```python
from build123d import *

# Parameters (mm, degrees)
CYLINDER016_R     = 2
CYLINDER016_DEPTH = 94
CYLINDER030_R     = 2
CYLINDER030_DEPTH = 10
CYLINDER029_R     = 2
CYLINDER029_DEPTH = 10
CYLINDER001_W     = 10
CYLINDER001_H     = 5
CYLINDER001_ANGLE = 90
BOX002_W          = 10
BOX002_H          = 54
BOX002_DEPTH      = 11
BOX001_W          = 10
BOX001_H          = 62
BOX001_DEPTH      = 11
BOX_W             = 10
BOX_H             = 72
BOX_DEPTH         = 25
CYLINDER_W        = 10
CYLINDER_H        = 5
CYLINDER_ANGLE    = 90
CYLINDER017_W     = 10
CYLINDER017_H     = 87
CYLINDER017_ANGLE = 90
BOX004_W          = 25
BOX004_H          = 72
BOX004_DEPTH      = 15


with BuildPart() as obj1:
    # Cylinder016 → Cylinder016 (new body)
    with BuildSketch(Plane(origin=(6, -47.35, 51), x_dir=(1, 0, 0), z_dir=(0, 1, 0))):
        Circle(CYLINDER016_R)
    extrude(amount=CYLINDER016_DEPTH)


with BuildPart() as m3cuts003:
    # Cylinder030 → Cylinder030 (new body)
    with BuildSketch(Plane(origin=(5, 9, 70), x_dir=(1, 0, 0), z_dir=(0, 0, 1))):
        Circle(CYLINDER030_R)
    extrude(amount=CYLINDER030_DEPTH)


with BuildPart() as m3cute001:
    # Cylinder029 → Cylinder029 (new body)
    with BuildSketch(Plane(origin=(5, -9, 70), x_dir=(1, 0, 0), z_dir=(0, 0, 1))):
        Circle(CYLINDER029_R)
    extrude(amount=CYLINDER029_DEPTH)

    # Fusion012: union m3Cuts003
    add(m3cuts003.part)


with BuildPart() as m3cute001_1:
    # Fusion012 placement: moved
    add(m3cute001.part.moved(Location((0, 0, -5))))


with BuildPart() as cylinder001:
    # Cylinder001 → Cylinder001 (revolve)
    with BuildSketch(Plane(origin=(10, -31, 55), x_dir=(-1, 0, 0), z_dir=(0, 0, 1))):
        with Locations((5, 2.5)):
            Rectangle(CYLINDER001_W, CYLINDER001_H)
    revolve(axis=Axis((10, -31, 55), (0, -1, 0)), revolution_arc=CYLINDER001_ANGLE)


with BuildPart() as in001:
    # Box002 → Box002 (new body)
    with BuildSketch(Plane(origin=(0, -27, 45), x_dir=(1, 0, 0), z_dir=(0, 0, 1))):
        with Locations((5, 27)):
            Rectangle(BOX002_W, BOX002_H)
    extrude(amount=BOX002_DEPTH)


with BuildPart() as in002:
    # Box001 → Box001 (new body)
    with BuildSketch(Plane(origin=(0, -31, 54), x_dir=(1, 0, 0), z_dir=(0, 0, 1))):
        with Locations((5, 31)):
            Rectangle(BOX001_W, BOX001_H)
    extrude(amount=BOX001_DEPTH)

    # Fusion: union in001
    add(in001.part)


with BuildPart() as cut:
    # Box → Box (new body)
    with BuildSketch(Plane(origin=(0, -36, 45), x_dir=(1, 0, 0), z_dir=(0, 0, 1))):
        with Locations((5, 36)):
            Rectangle(BOX_W, BOX_H)
    extrude(amount=BOX_DEPTH)

    # Cut: cut in002
    add(in002.part, mode=Mode.SUBTRACT)


with BuildPart() as lowbase:
    # Cylinder → Cylinder (revolve)
    with BuildSketch(Plane(origin=(10, 31, 55), x_dir=(0, 0, -1), z_dir=(1, 0, 0))):
        with Locations((5, 2.5)):
            Rectangle(CYLINDER_W, CYLINDER_H)
    revolve(axis=Axis((10, 31, 55), (0, 1, 0)), revolution_arc=CYLINDER_ANGLE)

    # Fusion001: union Cylinder001, Cut
    add(cylinder001.part)
    add(cut.part)

    # Cut003: cut m3Cute001
    add(m3cute001_1.part, mode=Mode.SUBTRACT)

    # Cut004: cut obj1
    add(obj1.part, mode=Mode.SUBTRACT)


with BuildPart() as include001:
    # Cylinder017 → Cylinder017 (revolve)
    with BuildSketch(Plane(origin=(10, -40.75, 55), x_dir=(0, 0, -1), z_dir=(1, 0, 0))):
        with Locations((5, 43.5)):
            Rectangle(CYLINDER017_W, CYLINDER017_H)
    revolve(axis=Axis((10, -40.75, 55), (0, 1, 0)), revolution_arc=CYLINDER017_ANGLE)


with BuildPart() as common:
    # Box004 → Box004 (new body)
    with BuildSketch(Plane(origin=(-15, -36, 55), x_dir=(1, 0, 0), z_dir=(0, 0, 1))):
        with Locations((12.5, 36)):
            Rectangle(BOX004_W, BOX004_H)
    extrude(amount=BOX004_DEPTH)

    # Fusion014: union include001
    add(include001.part)

    # Common: intersect lowBase
    add(lowbase.part, mode=Mode.INTERSECT)


solid = common.part
```
Here's how the part is built. I have some questions about the finished solid (model axes, mm). A direction names the side the tool comes from. Give positions to 0.01 mm unless a question says otherwise; leave off trailing zeros. Order: outer loops, then holes, each group sorted by start corner. A loop starts at its lowest first (then second) coordinate and runs counter-clockwise, first axis right, second up. Notation, with made-up numbers: (-14, 89) -> (44, 89) arc R29 cw to (44, 116) -> close; hole circle Ø2 at (21, -29). An arc over 180 degrees is marked (long way). Use CSV: the item, a comma, the result in double quotes. Start each with the question number.
Item 1: If I drill on probe 1 along Y at (x, z) = (5, 68.25); probe 2 along Y at (x, z) = (6.5, 60.25); probe 3 along Y at (x, z) = (9.75, 47.75), over which ranges is the centre line in solid material (lowest first)? Write a range as [from, to].
Item 2: Suppose I cut it at D-D (x = 2). List the corners of the cut face in (y, z) for me.
Item 3: On a 3-axis mill with a long thin cutter (end or side, diameter ignored), from which of +Z, -Z, +X, -X, +Y, -Y can I reach the whole of each face in a straight line? I mean faces 5 (the flat face through (5, 31, 59)), 6 (the flat face through (6, 27, 48)), 7 (the cylindrical face through (3.01, -31.44, 47.85)). Say none if no direction works.
Item 4: Suppose I cut it at A-A (x = 5). List the corners of the cut face in (y, z) for me.
Item 5: Suppose I cut it at B-B (z = 47.25). List the corners of the cut face in (x, y) for me, and give its area (3 significant figures).
Item 6: Suppose I cut it at C-C (y = -9). List the corners of the cut face in (x, z) for me.
Item 7: I'm going to push a flat-ended pin straight in: P1, Ø5, axis at x = 5, y = 9, coming from the -Z side. Where does the tip first touch, or does it pass through?
Item 8: Thinking about a two-plate mould opening in Y: for faces 1 (the flat face through (5, 29, 54)), 2 (the flat face through (6, -27, 48)), 3 (the flat face through (5, -36, 57)), 4 (the cylindrical face through (6, 31, 53)), which applies, pulls with the +Y half, pulls with the -Y half, needs draft (parallel to the pull), parting line crosses it, or undercut?
Answer block:
1,probe 1,"y = [-36, -11], [-7, 7], [11, 36]"
1,probe 2,"y = [-36, -31], [31, 36]"
1,probe 3,"y = [-36, -27], [27, 36]"
2,outline,"(-36, 49) -> (-27, 49) -> (-27, 54) -> (-31, 54) -> (-31, 65) -> (31, 65) -> (31, 54) -> (27, 54) -> (27, 49) -> (36, 49) -> (36, 70) -> (-36, 70) -> close"
3,face 5,"+X, -X"
3,face 6,"-Z, +X, -X"
3,face 7,"-Z, -X, +Y, -Y"
4,outline,"(-36, 46.34) -> (-27, 46.34) -> (-27, 49.27) -> (-36, 49.27) -> close; (-36, 52.73) -> (-27, 52.73) -> (-27, 54) -> (-31, 54) -> (-31, 65) -> (-11, 65) -> (-11, 70) -> (-36, 70) -> close; (-7, 65) -> (7, 65) -> (7, 70) -> (-7, 70) -> close; (11, 65) -> (31, 65) -> (31, 54) -> (27, 54) -> (27, 52.73) -> (36, 52.73) -> (36, 70) -> (11, 70) -> close; (27, 46.34) -> (36, 46.34) -> (36, 49.27) -> (27, 49.27) -> close"
5,outline,"(3.68, -36) -> (10, -36) -> (10, -27) -> (3.68, -27) -> close; (3.68, 27) -> (10, 27) -> (10, 36) -> (3.68, 36) -> close"
5,area,"114 mm^2"
6,outline,"(0, 65) -> (3, 65) -> (3, 70) -> (0, 70) -> close; (7, 65) -> (10, 65) -> (10, 70) -> (7, 70) -> close"
7,P1,"stops at z = 65"
8,face 1,"undercut"
8,face 2,"undercut"
8,face 3,"pulls with the -Y half"
8,face 4,"needs draft"
